Geometry check sheet. Reference: the model listing, model coordinates, mm. A direction names the side the tool comes from. Round coordinates to 2 decimals unless told otherwise and drop trailing zeros. Loops run counter-clockwise (first coordinate to the right, second up) from the corner with the lowest first, then second, coordinate; pieces in that order, holes last. Notation, with made-up numbers: (49.25, 6) - (82.25, 6) arc R15 cw to (82.25, 19) - close; hole circle Ø4 at (76.25, -17). An arc over 180 degrees is marked (long way). Answer as CSV lines item,"result". Start each with the question number.
1) Cross-section at A-A on y = 143. Record the boundary of the cut face in (x, z), and give its area (3 significant figures).
2) Access from +Z, -Z, +X, -X, +Y, -Y to the whole of each face (thin tool, end or side, straight path). Record for faces 1 (the cylindrical face through (214.142, 25.406, 40.214)), 2 (the flat face through (160.655, 100.889, 93.7)), 3 (the flat face through (63, 78, 25.4)), 4 (the flat face through (232.5, 100.89, 21.86)).
3) Cross-section at B-B on y = 101.6. Record the boundary of the cut face in (x, z), and give its area (3 significant figures).
4) Depth check by flat-ended pin: P1, Ø2, axis at y = 48, z = 71.5, coming from the +X side; P2, Ø1.5, axis at x = 198, y = 42.5, coming from the +Z side; P3, Ø12, axis at y = 108.5, z = 106, coming from the -X side. Enter the tip coordinate at first touch or a pass-through.
5) Draft check along Y on faces 5 (the flat face through (145, 203.2, 54)), 6 (the flat face through (219.8, 100.2, 8.8)), 7 (the flat face through (145, 0, 54)), 8 (the flat face through (25, 76.2, 13)). Enter one of: released by +Y, released by -Y, zero draft, split by the parting line, or undercut.
6) Cross-section at C-C on y = 189.5. Record the boundary of the cut face in (x, z), and give its area (3 significant figures).
7) Thickness scan on line 1 along Z through (x, y) = (135.5, 102.5); line 2 along X through (y, z) = (9.5, 25.5); line 3 along X through (y, z) = (55, 19.5). Record the ranges inside material, lowest first.
8) Cross-section at D-D on z = 39. State how many separate pieces and enclosed holes the cut face has, and give its area (3 significant figures).
from build123d import *

# Parameters (mm, degrees)
F1_DEPTH = 203.2
F3_DEPTH = 38.1
F5_DEPTH = 50.8


with BuildPart() as f1:
    # F0 (on Front) → F1 (new body)
    with BuildSketch(Plane.XZ):
        Polygon((0, 25.4), (0, 0), (127, 0), (177.8, 50.8), (228.6, 0), (254, 25.4), (128.276414, 151.123586), (102.876414, 125.723586), (152.4, 76.2), (101.6, 25.4), align=None)
    extrude(amount=-F1_DEPTH)

    # F2 (on face) → F3 (cut)
    with BuildSketch(Plane.XY.offset(25.4)):
        with BuildLine():
            Line((0, 76.2), (50.8, 76.2))
            ThreePointArc((50.8, 76.2), (76.2, 101.6), (50.8, 127))
            Line((50.8, 127), (0, 127))
            Line((0, 127), (0, 76.2))
        make_face()
    extrude(amount=-F3_DEPTH, mode=Mode.SUBTRACT)

    # F4 (on face) → F5 (cut)
    with BuildSketch(Plane(origin=(139.7, 0, 139.7), x_dir=(0.707107, 0, -0.707107), z_dir=(0.707107, 0, 0.707107))):
        with BuildLine():
            Line((-3.45539, 152.4), (-3.45539, 50.8))
            ThreePointArc((-3.45539, 50.8), (21.94461, 25.4), (47.34461, 50.8))
            Line((47.34461, 50.8), (47.34461, 152.4))
            ThreePointArc((47.34461, 152.4), (21.94461, 177.8), (-3.45539, 152.4))
        make_face()
        with BuildLine():
            Line((98.14461, 152.4), (98.14461, 50.8))
            ThreePointArc((98.14461, 50.8), (123.54461, 25.4), (148.94461, 50.8))
            Line((148.94461, 50.8), (148.94461, 152.4))
            ThreePointArc((148.94461, 152.4), (123.54461, 177.8), (98.14461, 152.4))
        make_face()
    extrude(amount=-F5_DEPTH, mode=Mode.SUBTRACT)


solid = f1.part
Answer block:
1,outline,"(0, 0) - (127, 0) - (177.8, 50.8) - (183.7, 44.9) - (209.1, 70.3) - (173.18, 106.22) - (147.78, 80.82) - (152.4, 76.2) - (101.6, 25.4) - (0, 25.4) - close; (102.88, 125.72) - (111.86, 116.74) - (137.26, 142.14) - (128.28, 151.12) - close; (219.62, 8.98) - (228.6, 0) - (254, 25.4) - (245.02, 34.38) - close"
1,area,"8,220 mm^2"
2,face 1,"none"
2,face 2,"+Z, -X"
2,face 3,"+Z, -X, +Y, -Y"
2,face 4,"+Z"
3,outline,"(76.2, 0) - (127, 0) - (177.8, 50.8) - (183.7, 44.9) - (209.1, 70.3) - (173.18, 106.22) - (147.78, 80.82) - (152.4, 76.2) - (101.6, 25.4) - (76.2, 25.4) - close; (102.88, 125.72) - (111.86, 116.74) - (137.26, 142.14) - (128.28, 151.12) - close; (219.62, 8.98) - (228.6, 0) - (254, 25.4) - (245.02, 34.38) - close"
3,area,"6,290 mm^2"
4,P1,"stops at x = 208.9"
4,P2,"stops at z = 82.15"
4,P3,"stops at x = 166.96"
5,face 5,"released by +Y"
5,face 6,"zero draft"
5,face 7,"released by -Y"
5,face 8,"undercut"
6,outline,"(0, 0) - (127, 0) - (177.8, 50.8) - (228.6, 0) - (254, 25.4) - (128.28, 151.12) - (102.88, 125.72) - (152.4, 76.2) - (101.6, 25.4) - (0, 25.4) - close"
6,area,"11,900 mm^2"
7,line 1,"z = 8.5 to 59.3, 140.39 to 143.9"
7,line 2,"x = 101.7 to 152.5, 203.1 to 253.9"
7,line 3,"x = 0 to 146.5, 230.14 to 248.1"
8,separate pieces,"3"
8,enclosed holes,"0"
8,area,"13,100 mm^2"
